Read the model definition and answer for the solid it produces. Units are mm, in the model's axes. Face numbers are marked on the shaded views. Coordinates: 2 decimals unless noted, no trailing zeros. Loops run counter-clockwise (first coordinate to the right, second up) from the corner with the lowest first, then second, coordinate; pieces in that order, holes last. Notation, with made-up numbers: (88.5, -34.5) -> (129.5, -34.5) arc R32 cw to (129.5, -8.5) -> close; hole circle Ø1 at (57, 58). An arc over 180 degrees is marked (long way). Answer as a JSON object with one key per item and string values. Group by question number.
Q1. The part is cut by section C-C on y = 22.5. Write down the section's boundary in (x, z), and give its area (3 significant figures).
Q2. This flat-tipped pin is pushed along its axis until it touches: P1, Ø8, axis at x = -24, y = -24, coming from the -Z side. Where does it stop, or does it pass through?
Q3. Determine the mould class of the marked faces 1, 2 and 3 for opening direction X: released by +X, released by -X, zero draft, split by the parting line, or undercut.
Q4. The part is cut by section A-A on x = 24. Write down the section's boundary in (y, z), and give its area (3 significant figures).
Q5. The part is cut by section B-B on z = 2.2. Write down the section's boundary in (x, y) (3 decimals), and give its area (3 significant figures).
Q6. Straight lines are drawn through the part: line 1 along Y through (x, z) = (24, 3.75); line 2 along Y through (x, z) = (-24.5, 3.9); line 3 along Y through (x, z) = (0, 2.2) (3 decimals). For each, find the intervals that lie inside material, in ascending order. Write a range as [from, to].
Q7. The part is cut by section D-D on y = 1. Write down the section's boundary in (x, z), and give its area (3 significant figures).
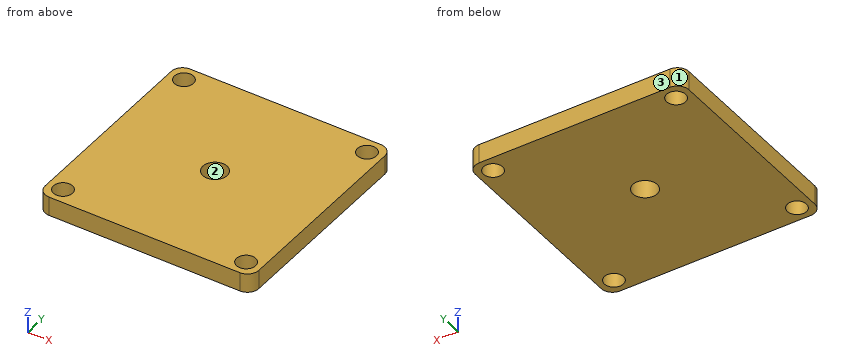
from build123d import *

# Parameters (mm, degrees)
SKETCH1_R           = 2.5
SKETCH1_R_2         = 3.175
BOSS_EXTRUDE1_DEPTH = 5


with BuildPart() as part:
    # Sketch1 → Boss-Extrude1 (new body)
    with BuildSketch(Plane.XY):
        with BuildLine():
            Line((-28, 25), (-28, -25))
            ThreePointArc((-28, -25), (-27.121320344, -27.121320344), (-25, -28))
            Line((-25, -28), (25, -28))
            ThreePointArc((25, -28), (27.121320344, -27.121320344), (28, -25))
            Line((28, -25), (28, 25))
            ThreePointArc((28, 25), (27.121320344, 27.121320344), (25, 28))
            Line((25, 28), (-25, 28))
            ThreePointArc((-25, 28), (-27.121320344, 27.121320344), (-28, 25))
        make_face()
        with Locations((-24, -24)):
            Circle(SKETCH1_R, mode=Mode.SUBTRACT)
        with Locations((24, -24)):
            Circle(SKETCH1_R, mode=Mode.SUBTRACT)
        with Locations((-24, 24)):
            Circle(SKETCH1_R, mode=Mode.SUBTRACT)
        Circle(SKETCH1_R_2, mode=Mode.SUBTRACT)
        with Locations((24, 24)):
            Circle(SKETCH1_R, mode=Mode.SUBTRACT)
    extrude(amount=BOSS_EXTRUDE1_DEPTH)


solid = part.part
Final values:
{
 "1": {"outline": "(-28, 0) -> (-26, 0) -> (-26, 5) -> (-28, 5) -> close; (-22, 0) -> (22, 0) -> (22, 5) -> (-22, 5) -> close; (26, 0) -> (28, 0) -> (28, 5) -> (26, 5) -> close", "area": "240 mm2"},
 "2": {"P1": "stops at z = 0"},
 "3": {"face 1": "released by -X", "face 2": "undercut", "face 3": "zero draft"},
 "4": {"outline": "(-28, 0) -> (-26.5, 0) -> (-26.5, 5) -> (-28, 5) -> close; (-21.5, 0) -> (21.5, 0) -> (21.5, 5) -> (-21.5, 5) -> close; (26.5, 0) -> (28, 0) -> (28, 5) -> (26.5, 5) -> close", "area": "230 mm2"},
 "5": {"outline": "(-28, -25) arc R3 ccw to (-25, -28) -> (25, -28) arc R3 ccw to (28, -25) -> (28, 25) arc R3 ccw to (25, 28) -> (-25, 28) arc R3 ccw to (-28, 25) -> close; hole circle Ø5 at (-24, -24); hole circle Ø5 at (-24, 24); hole circle Ø6.35 at (0, 0); hole circle Ø5 at (24, -24); hole circle Ø5 at (24, 24)", "area": "3,020 mm2"},
 "6": {"line 1": "y = [-28, -26.5], [-21.5, 21.5], [26.5, 28]", "line 2": "y = [-28, -26.45], [-21.55, 21.55], [26.45, 28]", "line 3": "y = [-28, -3.175], [3.175, 28]"},
 "7": {"outline": "(-28, 0) -> (-3.01, 0) -> (-3.01, 5) -> (-28, 5) -> close; (3.01, 0) -> (28, 0) -> (28, 5) -> (3.01, 5) -> close", "area": "250 mm2"}
}
